Build history of the part. All positions in model axes, mm. Face numbers are marked on the shaded views. A direction names the side the tool comes from. Round coordinates to 2 decimals unless told otherwise and drop trailing zeros. Write each loop counter-clockwise with the first axis right and the second up, starting at its lowest first coordinate (ties: lowest second). Pieces come first, ordered by that corner, then holes. Notation, with made-up numbers: (49.25, 50.5) -> (54.25, 50.5) arc R15 ccw to (54.25, 76.5) -> close; hole circle Ø4 at (-4.75, 10). An arc over 180 degrees is marked (long way). One line per question, with ' | ' between items.
from build123d import *

# Parameters (mm, degrees)
EXTRUDE_START                        = 16
EXTRUDE_1_DEPTH                      = 34
CHAMFER_1_SIZE                       = 2
PATTERN_CIRCULAR_1_COUNT             = 13
CHAMFER_1_OF_PATTERN_CIRCULAR_1_SIZE = 2
CUT_EXTRUDE_1_DEPTH                  = 2.5


with BuildPart() as part:
    # Эскиз1 → Повернуть1 (revolve)
    with BuildSketch(Plane(origin=(0, 0, 0), x_dir=(0, 0, -1), z_dir=(1, 0, 0)), mode=Mode.PRIVATE) as revolve_1_sk:
        Polygon((84.551755586, 0), (84.551755586, 7), (83.551755586, 8.5), (74.551755586, 8.5), (72.551755586, 8), (70.551755586, 8), (70.551755586, 9), (50.551755586, 9), (50.551755586, 8), (47.551755586, 8), (47.551755586, 10), (20.551755586, 10), (20.551755586, 9), (17.551755586, 9), (17.551755586, 10), (-16.448244414, 10), (-16.448244414, 9), (-19.448244414, 9), (-19.448244414, 10), (-55.448244414, 10), (-57.448244414, 8), (-57.448244414, 0), align=None)
    revolve(revolve_1_sk.sketch.rotate(Axis((0, 0, 57.448244414), (0, 0, -1)), 90), axis=Axis((0, 0, 57.448244414), (0, 0, -1)))

    # Эскиз2 → Бобышка-Вытянуть1 (add)
    with BuildSketch(Plane.XY.offset(0.448244414).offset(EXTRUDE_START)):
        with BuildLine():
            Line((1.566976519, 9.876466199), (1.566976519, 12.905215403))
            Line((1.566976519, 12.905215403), (0.993843905, 14.967039597))
            ThreePointArc((0.993843905, 14.967039597), (0, 15), (-0.993843905, 14.967039597))
            Line((-0.993843905, 14.967039597), (-1.566976519, 12.905215403))
            Line((-1.566976519, 12.905215403), (-1.566976519, 9.876466199))
            ThreePointArc((-1.566976519, 9.876466199), (0, 10), (1.566976519, 9.876466199))
        make_face()
    extrude_1 = extrude(amount=-EXTRUDE_1_DEPTH)

    # Фаска1
    chamfer_1_edges = [part.edges().sort_by_distance(p)[0] for p in [
        (0, 15, 16.448244414),
        (0, 15, -17.551755586),
    ]]
    chamfer(chamfer_1_edges, length=CHAMFER_1_SIZE)

    # Круговой массив1: Бобышка-Вытянуть1 ×13 about axis
    pattern_circular_1_axis = Axis((0, 0, 0), (0, 0, 1))
    for i in range(1, PATTERN_CIRCULAR_1_COUNT):
        add(extrude_1.rotate(pattern_circular_1_axis, i * 360 / PATTERN_CIRCULAR_1_COUNT))

    # Фаска1 of Круговой массив1
    chamfer_1_of_pattern_circular_1_edges = [part.edges().sort_by_distance(p)[0] for p in [
        (-6.970847581, 13.281840385, 16.448244414),
        (-6.970847581, 13.281840385, -17.551755586),
        (-12.344757988, 8.520971201, 16.448244414),
        (-12.344757988, 8.520971201, -17.551755586),
        (-14.890633111, 1.808050204, 16.448244414),
        (-14.890633111, 1.808050204, -17.551755586),
        (-14.02524364, -5.319073306, 16.448244414),
        (-14.02524364, -5.319073306, -17.551755586),
        (-9.946839874, -11.227661223, 16.448244414),
        (-9.946839874, -11.227661223, -17.551755586),
        (-3.589734964, -14.564127261, 16.448244414),
        (-3.589734964, -14.564127261, -17.551755586),
        (3.589734964, -14.564127261, 16.448244414),
        (3.589734964, -14.564127261, -17.551755586),
        (9.946839874, -11.227661223, 16.448244414),
        (9.946839874, -11.227661223, -17.551755586),
        (14.02524364, -5.319073306, 16.448244414),
        (14.02524364, -5.319073306, -17.551755586),
        (14.890633111, 1.808050204, 16.448244414),
        (14.890633111, 1.808050204, -17.551755586),
        (12.344757988, 8.520971201, 16.448244414),
        (12.344757988, 8.520971201, -17.551755586),
        (6.970847581, 13.281840385, 16.448244414),
        (6.970847581, 13.281840385, -17.551755586),
    ]]
    chamfer(chamfer_1_of_pattern_circular_1_edges, length=CHAMFER_1_OF_PATTERN_CIRCULAR_1_SIZE)

    # Эскиз3 → Вырез-Вытянуть1 (cut, symmetric)
    with BuildSketch(Plane(origin=(0, 0, 0), x_dir=(0, 0, -1), z_dir=(1, 0, 0))):
        with BuildLine():
            Line((51.264667775, 10.5), (69.838843396, 10.5))
            ThreePointArc((69.838843396, 10.5), (60.551755586, 3), (51.264667775, 10.5))
        make_face()
    extrude(amount=CUT_EXTRUDE_1_DEPTH, both=True, mode=Mode.SUBTRACT)


solid = part.part
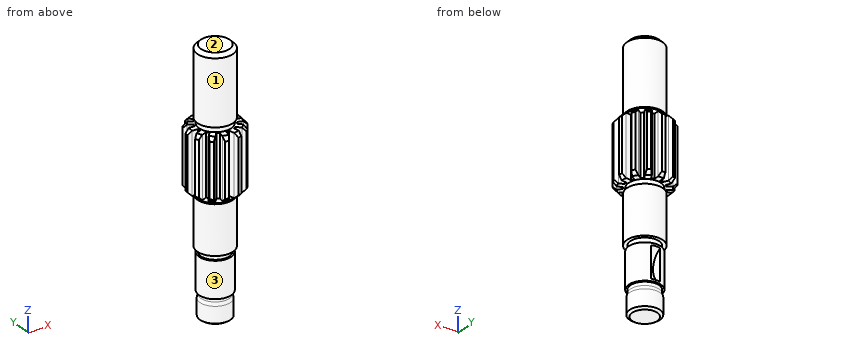
(1) 3-axis set-ups, long thin cutter, end or side, ignore diameter. For the marked faces 1, 2 and 3: which of +Z, -Z, +X, -X, +Y, -Y reach the whole face in a straight line?
Calculated:
face 1: +Z | face 2: +Z, +X, -X, +Y, -Y | face 3: -Z
(2) Slice it at A-A (z = -28). Write the cut outline in (x, y).
Calculated:
outline: circle Ø20 at (0, 0)
(3) Drop flat-ended pins along their axis: pin 1 (12 mm diameter, centred on x = 1, z = 23, fed in from +Y); pin 2 (2 mm diameter, centred on y = -4.5, z = 32, fed in from +X); pin 3 (4.5 mm diameter, centred on y = 6.5, z = -60.5, fed in from +X); pin 4 (5 mm diameter, centred on x = -1.5, z = 9.5, fed in from +Y). Give the stop position or say it passes through.
Calculated:
pin 1: y = 10 | pin 2: x = 9.37 | pin 3: x = 7.93 | pin 4: y = 15
(4) Wall check: line 1 (X direction, y = 10.5, z = 5); line 2 (Y direction, x = 10.5, z = 4); line 3 (Z direction, x = -1, y = 9.75). Give the ranges that are in metal, low to high. Write a range as from..to.
Calculated:
line 1: -7.28..-3.74, -1.57..1.57, 3.74..7.28 | line 2: -10.71..-10.2, -5.66..-2.31, -0.3..2.85, 5.34..8.89 | line 3: -47.55..-20.55, -17.55..16.45, 19.45..55.65
